from build123d import *

# Parameters (mm, degrees)
BODY_DEPTH   = 9
SK_HOLE_V_R  = 4
HOLE_V_DEPTH = 59.071077138


with BuildPart() as part:
    # sk-body → body (new, symmetric)
    with BuildSketch(Plane.XY):
        Polygon((-13.5, 28.4), (0, 28.4), (0, -15), (-13.5, -15), (-13.5, 0), (-49.5, 0), (-49.5, 14), (-13.5, 14), align=None)
    extrude(amount=BODY_DEPTH, both=True)

    # sk-hole_v → hole_v (cut, through all)
    with BuildSketch(Plane(origin=(0, 14, 0), x_dir=(-1, 0, 0), z_dir=(0, 1, 0))):
        with Locations(Location((40.5, 0, 0), (0, 0, 90))):
            Circle(SK_HOLE_V_R)
        with Locations(Location((23.5, 0, 0), (0, 0, 90))):
            Circle(SK_HOLE_V_R)
    extrude(amount=-HOLE_V_DEPTH, mode=Mode.SUBTRACT)


solid = part.part
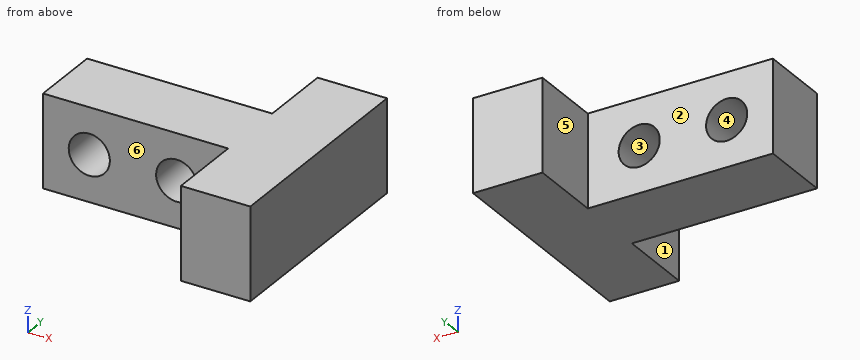
Model file for the job. Use its own axes, mm. Face numbers are marked on the shaded views. A direction names the side the tool comes from. Give positions to 0.01 mm unless a question says otherwise; leave off trailing zeros. Order: outer loops, then holes, each group sorted by start corner. A loop starts at its lowest first (then second) coordinate and runs counter-clockwise, first axis right, second up. Notation, with made-up numbers: M -9.5,-25.5 L 48.5,-25.5 A33 cw 48.5,5.5 Z; hole C -1.5,27.25 d10. An arc over 180 degrees is marked long. Put each result on its own line as item: value. Start each with the question number.
(1) Pin check, flat tips, straight feed: pin 1 Ø9 at (x, z) = (-36.5, -3.5) entering from -Y; pin 2 Ø12 at (x, y) = (-30, 17.5) entering from -Z; pin 3 Ø7.5 at (y, z) = (-7.5, -3.5) entering from -X; pin 4 Ø9 at (x, z) = (-40.5, 0) entering from +Y. Stop position of each tip, or through.
(2) Band-saw the part on D-D on z = -7.25. Give the cut face in (x, y), then the cut area to 3 significant figures.
(3) Pull direction X, two halves, no side cores. Call the marked faces 4, 5 and 6: released by +X, released by -X, zero draft, split by the parting line, or undercut.
(4) Band-saw the part on B-B on z = 0. Give the cut face in (x, y).
(5) Tool access for the marked faces 1, 2 and 3: list every direction of +Z, -Z, +X, -X, +Y, -Y with a clear straight run to the whole face (end or side of a thin tool).
(6) Band-saw the part on A-A on x = -23.5. Give the cut face in (y, z), then the cut area to 3 significant figures.
(7) Drill centre lines: L1, parallel to X at y = 5.75, z = 0; L2, parallel to Y at x = -16.5, z = -2.75; L3, parallel to X at y = 3.5, z = 1. Where is each one in solid material? Low to high. Write a range as [from, to].
(8) Band-saw the part on C-C on y = 12. Give the cut face in (x, z), then the cut area to 3 significant figures.
Results below:
1. pin 1: stops at y = 0
1. pin 2: stops at z = -9
1. pin 3: stops at x = -13.5
1. pin 4: stops at y = 14
2. outline: M -49.5,0 L -13.5,0 L -13.5,-15 L 0,-15 L 0,28.4 L -13.5,28.4 L -13.5,14 L -49.5,14 Z
2. area: 1,090 mm2
3. face 4: undercut
3. face 5: released by -X
3. face 6: zero draft
4. outline: M -49.5,0 L -44.5,0 L -44.5,14 L -49.5,14 Z; M -36.5,0 L -27.5,0 L -27.5,14 L -36.5,14 Z; M -19.5,0 L -13.5,0 L -13.5,-15 L 0,-15 L 0,28.4 L -13.5,28.4 L -13.5,14 L -19.5,14 Z
5. face 1: +Z, -Z, -X, -Y
5. face 2: +Z, -Z, -X, +Y
5. face 3: +Y, -Y
6. outline: M 0,-9 L 14,-9 L 14,-4 L 0,-4 Z; M 0,4 L 14,4 L 14,9 L 0,9 Z
6. area: 140 mm2
7. L1: x = [-49.5, -44.5], [-36.5, -27.5], [-19.5, 0]
7. L2: y = [0, 14]
7. L3: x = [-49.5, -44.37], [-36.63, -27.37], [-19.63, 0]
8. outline: M -49.5,-9 L 0,-9 L 0,9 L -49.5,9 Z; hole C -40.5,0 d8; hole C -23.5,0 d8
8. area: 790 mm2
